Source: CAD feature listing. Evaluate the final solid. Frame: model axes, mm. Round coordinates to 2 decimals unless told otherwise and drop trailing zeros. Write each loop counter-clockwise with the first axis right and the second up, starting at its lowest first coordinate (ties: lowest second). Pieces come first, ordered by that corner, then holes. Notation, with made-up numbers: M 45.25,30 L 71.25,30 A22 cw 71.25,41 Z; hole C 31.5,69 d4. An arc over 180 degrees is marked long. Put each result on its own line as item: value. Start each with the question number.
```python
from build123d import *

# Parameters (mm, degrees)
EXTRUDE_1_DEPTH   = 30
HOLE_WIZARD_M31_D = 2.5


with BuildPart() as part:
    # Эскиз1 → Бобышка-Вытянуть1 (new body)
    with BuildSketch(Plane(origin=(0, 0, 0), x_dir=(1, 0, 0), z_dir=(0, 1, 0))):
        Polygon((0, 2.886751346), (-2.5, 1.443375673), (-2.5, -1.443375673), (0, -2.886751346), (2.5, -1.443375673), (2.5, 1.443375673), align=None)
    extrude(amount=EXTRUDE_1_DEPTH)

    # Отверстие обработанное метчиком M31 (through all)
    with Locations(Plane(origin=(0, 30, 0), x_dir=(1, 0, 0), z_dir=(0, 1, 0))):
        with Locations((0, 0)):
            Hole(HOLE_WIZARD_M31_D / 2)

    # Эскиз4 → Вырез-Повернуть1 (revolve, cut)
    with BuildSketch(Plane(origin=(0, 0, 0), x_dir=(0, 0, -1), z_dir=(1, 0, 0)), mode=Mode.PRIVATE) as cut_revolve_1_sk:
        Polygon((1.86348431, 30.302108364), (3.639820408, 29.27654024), (3.639820408, 31.381488227), (1.86348431, 31.381488227), align=None)
        Polygon((1.86348431, -0.302108364), (3.639820408, 0.72345976), (3.639820408, -1.381488227), (1.86348431, -1.381488227), align=None)
    revolve(cut_revolve_1_sk.sketch.rotate(Axis((0, 0, 0), (0, 1, 0)), 180), axis=Axis((0, 0, 0), (0, 1, 0)), mode=Mode.SUBTRACT)


solid = part.part
```
(1) Contact query for flat-ended pins moving along their axis: P1, Ø3, axis at x = -1, z = 0.5, coming from the -Y side; P2, Ø1.5, axis at x = -0.5, y = 25.5, coming from the -Z side. Output: stop coordinate, or through.
(2) Section query A-A (z = 0). Return loops of the section in (x, y).
(3) Ray query, line 1 along X through (y, z) = (19.75, 0.05); line 2 along Z through (x, y) = (-0.2, 7.75); line 3 along X through (y, z) = (4.5, 1.1). Return the intervals inside material, ascending.
(4) Section query B-B (y = 17.25). Return loops of the section in (x, z), and give its area (3 significant figures).
Entries:
1. P1: y = 0
1. P2: z = -2.89
2. outline: M -2.5,0.07 L -2.39,0 L -1.25,0 L -1.25,30 L -2.39,30 L -2.5,29.93 Z; M 1.25,0 L 2.39,0 L 2.5,0.07 L 2.5,29.93 L 2.39,30 L 1.25,30 Z
3. line 1: -2.5 to -1.25, 1.25 to 2.5
3. line 2: -2.77 to -1.23, 1.23 to 2.77
3. line 3: -2.5 to -0.59, 0.59 to 2.5
4. outline: M -2.5,-1.44 L 0,-2.89 L 2.5,-1.44 L 2.5,1.44 L 0,2.89 L -2.5,1.44 Z; hole C 0,0 d2.5
4. area: 16.7 mm2
